Geometry: final body of the model. Coordinates: model frame, mm. A direction names the side the tool comes from. Give positions to 0.01 mm unless a question says otherwise; leave off trailing zeros. Order: outer loops, then holes, each group sorted by start corner. A loop starts at its lowest first (then second) coordinate and runs counter-clockwise, first axis right, second up. Notation, with made-up numbers: (-28.75, 29.5) -> (26.25, 29.5) arc R32 ccw to (26.25, 66.5) -> close; hole circle Ø9 at (-34.5, -40). An arc over 180 degrees is marked (long way). Answer in a Markdown table with one row per item. Add a question column.
Q1. Pull-direction query (Y, two-part tool) for faces 1 (the face through (-14, 0, 1)), 2 (the face through (23.5, 35, -1)), 3 (the face through (21.035, 55.751, -15.535)); classes: +Y half, -Y half, draft (parallel to the pull), parting line (faces both ways), or undercut.
Q2. Set-up query: faces 4 (the face through (-45, 38, -26.585)), 5 (the face through (0, 37, -83.75)), 6 (the face through (0, 30, 83.75)), 7 (the face through (-47, 2, 45.415)), 8 (the face through (-47, 37, 30.415)). Return all of +Z, -Z, +X, -X, +Y, -Y with unobstructed straight access to the full face (end or side cutting, diameter ignored); none if empty.
Q3. Cut plane B-B on x = -43.5. Return the cut outline in (y, z).
Q4. Cut plane C-C on z = -35.5. Return the cut outline in (x, y).
Q5. Line query: line 1 along X through (y, z) = (37, 38); line 2 along Z through (x, y) = (-36, 66); line 3 along X through (y, z) = (23.5, -12). Output: solid intervals per line, ascending. Write a range as from..to.
Q6. Cut plane A-A on y = 27.5. Return the cut outline in (x, z).
Q7. Cut plane D-D on y = 55. Count the separate pieces of the cut face and the enclosed holes in it, and give its area (3 significant figures).
Q8. Contact query for flat-ended pins moving along their axis: P1, Ø4.5, axis at x = -58, z = 34.5, coming from the +Y side; P2, Ø2, axis at x = 0, z = 91.38, coming from the +Y side; P3, Ø8, axis at x = 12, y = 29.5, coming from the +Z side; P4, Ø4, axis at x = -47, y = 14.5, coming from the -Z side. Output: stop coordinate, or through.
from build123d import *
from OCP.BRepFilletAPI import BRepFilletAPI_MakeChamfer

# Parameters (mm, degrees)
ESBO_O1_W                = 47
ESBO_O1_H                = 62
ESBO_O1_H_2              = 167.5
RESSALTO_EXTRUS_O1_DEPTH = 70
ESBO_O3_W                = 37
ESBO_O3_H                = 157.5
CORTE_EXTRUS_O2_DEPTH    = 65
ESBO_O5_W                = 37
ESBO_O5_H                = 31.934482306
CORTE_EXTRUS_O3_DEPTH    = 30
ESBO_O11_W               = 47
ESBO_O11_H               = 15
RESSALTO_EXTRUS_O2_DEPTH = 5
ESBO_O12_R               = 1.65
CORTE_EXTRUS_O6_DEPTH    = 138.647420971
ESBO_O14_R               = 2.5
CORTE_EXTRUS_O8_DEPTH    = 154.256525147
ESBO_O15_W               = 42
ESBO_O15_H               = 53
CORTE_EXTRUS_O10_DEPTH   = 65
CHANFRO9_SIZE            = 5
CHANFRO9_SIZE2           = 17.907987678


with BuildPart() as part:
    # Esboço1 → Ressalto-extrusão1 (new body)
    with BuildSketch(Plane(origin=(0, 0, 0), x_dir=(1, 0, 0), z_dir=(0, 1, 0))):
        with Locations((-47, 0.585067636)):
            Rectangle(ESBO_O1_W, ESBO_O1_H)
        Rectangle(ESBO_O1_W, ESBO_O1_H_2)
    extrude(amount=RESSALTO_EXTRUS_O1_DEPTH)

    # Esboço3 → Corte-extrusão2 (cut)
    with BuildSketch(Plane(origin=(0, 70, 0), x_dir=(1, 0, 0), z_dir=(0, 1, 0))):
        Rectangle(ESBO_O3_W, ESBO_O3_H)
    extrude(amount=-CORTE_EXTRUS_O2_DEPTH, mode=Mode.SUBTRACT)

    # Esboço5 → Corte-extrusão3 (cut)
    with BuildSketch(Plane(origin=(0, 70, 0), x_dir=(1, 0, 0), z_dir=(0, 1, 0))):
        with Locations((0, -78.75)):
            Rectangle(ESBO_O5_W, ESBO_O5_H)
    extrude(amount=-CORTE_EXTRUS_O3_DEPTH, mode=Mode.SUBTRACT)

    # Esboço11 → Ressalto-extrusão2 (add)
    with BuildSketch(Plane.XZ):
        with Locations((0, -91.25)):
            Rectangle(ESBO_O11_W, ESBO_O11_H)
        with Locations((0, 91.25)):
            Rectangle(ESBO_O11_W, ESBO_O11_H)
        with Locations((-47, -39.085067636)):
            Rectangle(ESBO_O11_W, ESBO_O11_H)
        with Locations((-47, 37.914932364)):
            Rectangle(ESBO_O11_W, ESBO_O11_H)
    extrude(amount=-RESSALTO_EXTRUS_O2_DEPTH)

    # Esboço12 → Corte-extrusão6 (cut, through all)
    with BuildSketch(Plane(origin=(0, 5, 0), x_dir=(1, 0, 0), z_dir=(0, 1, 0))):
        with Locations(Location((-47, -38.049932364, 0), (0, 0, 270))):
            Circle(ESBO_O12_R)
        with Locations(Location((-47, 39.215067636, 0), (0, 0, 270))):
            Circle(ESBO_O12_R)
        with Locations(Location((0, -91.38, 0), (0, 0, 270))):
            Circle(ESBO_O12_R)
        with Locations(Location((0, 91.38, 0), (0, 0, 270))):
            Circle(ESBO_O12_R)
    extrude(amount=-CORTE_EXTRUS_O6_DEPTH, mode=Mode.SUBTRACT)

    # Esboço14 → Corte-extrusão8 (cut, through all)
    with BuildSketch(Plane(origin=(23.5, 0, 0), x_dir=(0, 0, -1), z_dir=(1, 0, 0))):
        with Locations((-13.15, 55)):
            Circle(ESBO_O14_R)
        with Locations((13.15, 55)):
            Circle(ESBO_O14_R)
    extrude(amount=-CORTE_EXTRUS_O8_DEPTH, mode=Mode.SUBTRACT)

    # Esboço15 → Corte-extrusão10 (cut)
    with BuildSketch(Plane(origin=(0, 70, 0), x_dir=(1, 0, 0), z_dir=(0, 1, 0))):
        with Locations((-44.5, 0.085067636)):
            Rectangle(ESBO_O15_W, ESBO_O15_H)
    extrude(amount=-CORTE_EXTRUS_O10_DEPTH, mode=Mode.SUBTRACT)

    # Chanfro9: one chamfer whose edges measure the first distance from different faces: ONE call of the kernel's chamfer builder (chamfer() names one face for all edges)
    chanfro9_edges_1 = [part.edges().sort_by_distance(p)[0] for p in [
        (-23.5, 2.5, -98.75),
    ]]
    chanfro9_side_1 = [part.faces().sort_by_distance(p)[0] for p in [
        (-23.5, 35, -58.73896239),
    ]]
    chanfro9_edges_2 = [part.edges().sort_by_distance(p)[0] for p in [
        (23.5, 2.5, -98.75),
        (23.5, 2.5, 98.75),
    ]]
    chanfro9_side_2 = [part.faces().sort_by_distance(p)[0] for p in [
        (23.5, 34.521753359, 0),
    ]]
    chanfro9_edges_3 = [part.edges().sort_by_distance(p)[0] for p in [
        (-23.5, 2.5, 98.75),
    ]]
    chanfro9_side_3 = [part.faces().sort_by_distance(p)[0] for p in [
        (-23.5, 35, 58.153894753),
    ]]
    chanfro9 = BRepFilletAPI_MakeChamfer(part.part.solid().wrapped)
    for e in chanfro9_edges_1:
        chanfro9.Add(CHANFRO9_SIZE, CHANFRO9_SIZE2, e.wrapped, chanfro9_side_1[0].wrapped)  # the first distance lies on this face
    for e in chanfro9_edges_2:
        chanfro9.Add(CHANFRO9_SIZE, CHANFRO9_SIZE2, e.wrapped, chanfro9_side_2[0].wrapped)  # the first distance lies on this face
    for e in chanfro9_edges_3:
        chanfro9.Add(CHANFRO9_SIZE, CHANFRO9_SIZE2, e.wrapped, chanfro9_side_3[0].wrapped)  # the first distance lies on this face
    add(Compound.cast(chanfro9.Shape()), mode=Mode.REPLACE)


solid = part.part
Completed:
| question | item | result |
|---|---|---|
| 1 | face 1 | -Y half |
| 1 | face 2 | draft |
| 1 | face 3 | undercut |
| 2 | face 4 | +Y |
| 2 | face 5 | -Z, +X, -X, +Y |
| 2 | face 6 | +Z, +X, -X, +Y |
| 2 | face 7 | +Z, -X, +Y, -Y |
| 2 | face 8 | +Z, -X, +Y |
| 3 | outline | (0, -46.59) -> (5, -46.59) -> (5, -31.59) -> (70, -31.59) -> (70, -26.59) -> (5, -26.59) -> (5, 26.41) -> (70, 26.41) -> (70, 30.41) -> (5, 30.41) -> (5, 45.41) -> (0, 45.41) -> close |
| 4 | outline | (-70.5, 0) -> (23.5, 0) -> (23.5, 70) -> (18.5, 70) -> (18.5, 5) -> (-18.5, 5) -> (-18.5, 70) -> (-23.5, 70) -> (-23.5, 5) -> (-70.5, 5) -> close |
| 5 | line 1 | x = -23.5..-18.5, 18.5..23.5 |
| 5 | line 2 | z = -31.59..-26.59, 26.41..30.41 |
| 5 | line 3 | x = -70.5..-65.5, -23.5..-18.5, 18.5..23.5 |
| 6 | outline | (-70.5, -31.59) -> (-23.5, -31.59) -> (-23.5, -83.75) -> (23.5, -83.75) -> (23.5, 83.75) -> (-23.5, 83.75) -> (-23.5, 30.41) -> (-70.5, 30.41) -> close; hole (-65.5, -26.59) -> (-23.5, -26.59) -> (-23.5, 26.41) -> (-65.5, 26.41) -> close; hole (-18.5, -78.75) -> (18.5, -78.75) -> (18.5, 78.75) -> (-18.5, 78.75) -> close |
| 7 | separate pieces | 6 |
| 7 | enclosed holes | 0 |
| 7 | area | 2,400 mm² |
| 8 | P1 | stops at y = 5 |
| 8 | P2 | passes through |
| 8 | P3 | stops at z = 83.75 |
| 8 | P4 | stops at z = -31.59 |
